```python
from build123d import *

# Parameters (mm, degrees)
BOSS_EXTRUDE1_DEPTH = 3.5
SKETCH2_R           = 0.9
CUT_EXTRUDE1_DEPTH  = 75.183799012
SKETCH3_R           = 2.5
BOSS_EXTRUDE2_DEPTH = 10
SKETCH4_R           = 0.9
CUT_EXTRUDE2_DEPTH  = 10


with BuildPart() as part:
    # Sketch1 → Boss-Extrude1 (new body)
    with BuildSketch(Plane(origin=(0, 0, 0), x_dir=(1, 0, 0), z_dir=(0, 1, 0))):
        with BuildLine():
            Line((-21.702078291, 46.665350003), (-22.976238483, 49.381324194))
            ThreePointArc((-22.976238483, 49.381324194), (-16.705296787, 51.039340816), (-10.242062523, 50.491315514))
            ThreePointArc((-10.242062523, 50.491315514), (16.850294685, -49.735366194), (-21.702078291, 46.665350003))
        make_face()
    extrude(amount=BOSS_EXTRUDE1_DEPTH)

    # Sketch2 → Cut-Extrude1 (cut, through all)
    with BuildSketch(Plane(origin=(0, 3.5, 0), x_dir=(1, 0, 0), z_dir=(0, 1, 0))):
        with Locations(Location((-41.040664553, -16.531295011, 0), (0, 0, 270))):
            Circle(SKETCH2_R)
        with Locations(Location((39.259074256, 21.140171457, 0), (0, 0, 270))):
            Circle(SKETCH2_R)
    extrude(amount=-CUT_EXTRUDE1_DEPTH, mode=Mode.SUBTRACT)

    # Sketch3 → Boss-Extrude2 (add)
    with BuildSketch(Plane(origin=(0, 3.5, 0), x_dir=(1, 0, 0), z_dir=(0, 1, 0))):
        with Locations(Location((-22.661676127, 31.726346577, 0), (0, 0, 270))):
            Circle(SKETCH3_R)
        with Locations(Location((22.661676127, 31.726346577, 0), (0, 0, 270))):
            Circle(SKETCH3_R)
        with Locations(Location((22.661676127, -31.726346577, 0), (0, 0, 90))):
            Circle(SKETCH3_R)
        with Locations(Location((-22.661676127, -31.726346577, 0), (0, 0, 90))):
            Circle(SKETCH3_R)
    extrude(amount=BOSS_EXTRUDE2_DEPTH)

    # Sketch4 → Cut-Extrude2 (cut)
    with BuildSketch(Plane.XZ):
        with Locations(Location((18.995826683, 40.085484141, 0), (0, 0, 270))):
            Circle(SKETCH4_R)
    extrude(amount=-CUT_EXTRUDE2_DEPTH, mode=Mode.SUBTRACT)


solid = part.part
```
The model under review builds one solid part; all positions refer to its coordinate system, in mm. A direction names the side the tool comes from. Give positions to 0.01 mm unless a question says otherwise; leave off trailing zeros. Write each loop counter-clockwise with the first axis right and the second up, starting at its lowest first coordinate (ties: lowest second). Pieces come first, ordered by that corner, then holes.
(1) Tool access review of faces 4 (the flat face through (23, 13.5, -32)), 5 (the cylindrical face through (-22.552, 8.43, -34.224)): name each direction out of +Z, -Z, +X, -X, +Y, -Y from which nothing blocks a thin tool from reaching the whole face with its end or side.
(2) Consider section C-C, the plane x = -36.5. Give the boundary of the cut face in (y, z).
(3) The part is to be moulded in two halves that separate along X. For faces 1 (the cylindrical face through (-16.8, 1.73, -51.03)), 2 (the flat face through (1, 0, 0)), 3 (the flat face through (-22.33, 1.73, -48)), say which applies: released by +X, released by -X, zero draft, split by the parting line, or undercut.
(4) Consider section D-D, the plane z = -8.5. Give the boundary of the cut face in (x, y).
(5) To check wall thickness, follow L1, parallel to Y at x = 21, z = -18.5; L2, parallel to Z at x = 21, y = 6; L3, parallel to Z at x = 2, y = 1.25. State the ranges of each line that lie inside material, in increasing order.
(6) Consider section B-B, the plane y = 9.25. Give the boundary of the cut face in (x, z).
(7) Consider section A-A, the plane z = 31. Give the boundary of the cut face in (x, y).
(8) For P1, Ø3, axis at x = 39.26, z = -21.14, coming from the +Y side; P2, Ø2, axis at y = 2.5, z = -22, coming from the +X side; P3, Ø1.5, axis at y = 7, z = 30.5, coming from the +X side; P4, Ø1, axis at y = 11.5, z = 36, coming from the +X side, all flat-tipped, find the tip position at first contact; note any pin that passes through.
Returned:
1. face 4: +Z, -Z, +X, -X, +Y
1. face 5: +Y
2. outline: (0, -36.24) - (3.5, -36.24) - (3.5, 37.07) - (0, 37.07) - close
3. face 1: undercut
3. face 2: zero draft
3. face 3: released by -X
4. outline: (-50.85, 0) - (51.61, 0) - (51.61, 3.5) - (-50.85, 3.5) - close
5. L1: y = 0 to 3.5
5. L2: z = -33.59 to -29.86, 29.86 to 33.59
5. L3: z = -51.56 to 52.39
6. outline: circle Ø5 at (-22.66, -31.73); circle Ø5 at (-22.66, 31.73); circle Ø5 at (22.66, -31.73); circle Ø5 at (22.66, 31.73)
7. outline: (-41.67, 0) - (42.44, 0) - (42.44, 3.5) - (25.05, 3.5) - (25.05, 13.5) - (20.27, 13.5) - (20.27, 3.5) - (-20.27, 3.5) - (-20.27, 13.5) - (-25.05, 13.5) - (-25.05, 3.5) - (-41.67, 3.5) - close
8. P1: stops at y = 3.5
8. P2: stops at x = 47.77
8. P3: stops at x = 25.12
8. P4: passes through
